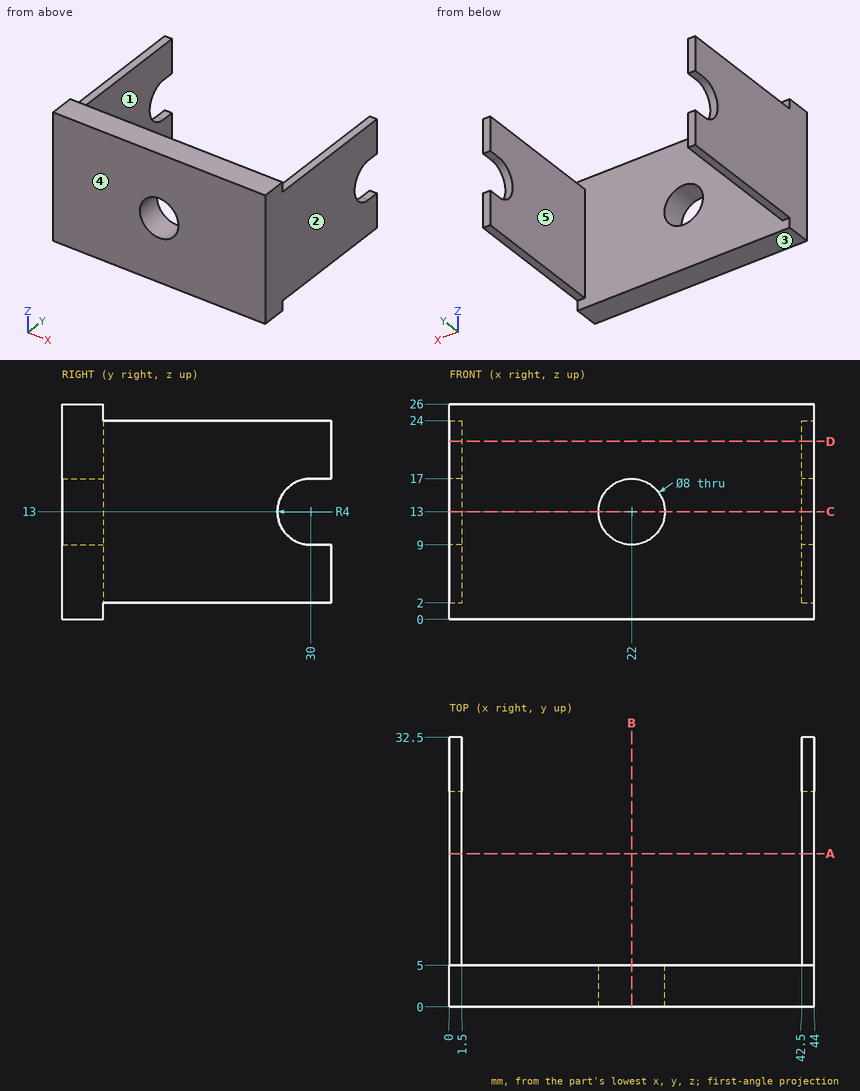
Input: dimensioned drawing with shaded views. Units: mm. Origin: part minimum x, y, z. A direction names the side the tool comes from. Coordinates: 2 decimals unless noted, no trailing zeros. Loops run counter-clockwise (first coordinate to the right, second up) from the corner with the lowest first, then second, coordinate; pieces in that order, holes last. Notation, with made-up numbers: (-36.5, -39) -> (7.5, -39) arc R15 cw to (7.5, -11) -> close; hole circle Ø8 at (58, 88). An arc over 180 degrees is marked (long way). One line per item, written item: value. Start each with the question number.
Q1. Section query D-D, the plane z = 21.5. Return the cut outline in (x, y), and give its area (4 significant figures).
Q2. Section query B-B, the plane x = 22. Return the cut outline in (y, z).
Q3. Set-up query: the marked faces 4 and 5. Return all of +Z, -Z, +X, -X, +Y, -Y with unobstructed straight access to the full face (end or side cutting, diameter ignored); none if empty.
Q4. Mould query, pull axis X, two halves, no side actions, for the marked faces 1, 2 and 3. Classes: pulls with the +X half, pulls with the -X half, needs draft (parallel to the pull), parting line crosses it, or undercut.
Q5. Section query A-A, the plane y = 18.5. Return the cut outline in (x, z), and give its area (3 significant figures).
Q6. Contact query for flat-ended pins moving along their axis: P1, Ø1.6, axis at x = 0.5, y = 21, coming from the +Z side; P2, Ø1.6, axis at x = 43.5, y = 24.5, coming from the -Z side; P3, Ø1.5, axis at x = 29.5, z = 22.5, coming from the +Y side. Output: stop coordinate, or through.
Q7. Section query C-C, the plane z = 13. Return the cut outline in (x, y), and give its area (3 significant figures).
Q8. Line query: line 1 along X through (y, z) = (24, 16.75); line 2 along Z through (x, y) = (22, 2.95); line 3 along Y through (x, z) = (36, 14.25). Output: solid intervals per line, ascending.
Results:
1. outline: (0, 0) -> (44, 0) -> (44, 32.5) -> (42.5, 32.5) -> (42.5, 5) -> (1.5, 5) -> (1.5, 32.5) -> (0, 32.5) -> close
1. area: 302.5 mm^2
2. outline: (0, 0) -> (5, 0) -> (5, 9) -> (0, 9) -> close; (0, 17) -> (5, 17) -> (5, 26) -> (0, 26) -> close
3. face 4: +Z, -Z, +X, -X, -Y
3. face 5: +Z, -Z, +Y
4. face 1: undercut
4. face 2: pulls with the +X half
4. face 3: needs draft
5. outline: (0, 2) -> (1.5, 2) -> (1.5, 24) -> (0, 24) -> close; (42.5, 2) -> (44, 2) -> (44, 24) -> (42.5, 24) -> close
5. area: 66.0 mm^2
6. P1: z = 24
6. P2: z = 2
6. P3: y = 5
7. outline: (0, 0) -> (18, 0) -> (18, 5) -> (1.5, 5) -> (1.5, 26) -> (0, 26) -> close; (26, 0) -> (44, 0) -> (44, 26) -> (42.5, 26) -> (42.5, 5) -> (26, 5) -> close
7. area: 243 mm^2
8. line 1: 0 to 1.5, 42.5 to 44
8. line 2: 0 to 9, 17 to 26
8. line 3: 0 to 5
